Can you work these out from the model? Positions are in its coordinate system, mm. Face numbers are marked on the shaded views. A direction names the side the tool comes from. Give positions to 0.01 mm unless a question says otherwise; leave off trailing zeros. Loops run counter-clockwise (first coordinate to the right, second up) from the corner with the lowest first, then second, coordinate; pieces in that order, holes last. Notation, with made-up numbers: (69, 65) - (122, 65) arc R20 cw to (122, 90) - close; hole circle Ø5 at (51.5, 12.25). An arc over 180 degrees is marked (long way). Answer in a Markdown table with one row per item.
from build123d import *

# Parameters (mm, degrees)
SKETCH_1_R          = 14
EXTRUDE_1_DEPTH     = 22
SKETCH_2_R          = 2.95
CUT_EXTRUDE_1_DEPTH = 1.1
SKETCH_3_R          = 2.6
CUT_EXTRUDE_2_DEPTH = 9
SKETCH_5_R          = 6.1
CUT_EXTRUDE_3_DEPTH = 11.9
SKETCH_6_R          = 7.05
CUT_EXTRUDE_4_DEPTH = 7.9
SKETCH_7_R          = 7.6
CUT_EXTRUDE_5_DEPTH = 3.9
SKETCH_8_R          = 11.75
CUT_EXTRUDE_6_DEPTH = 1.9


with BuildPart() as part:
    # Эскиз1 → Бобышка-Вытянуть1 (new body)
    with BuildSketch(Plane.XY):
        Circle(SKETCH_1_R)
    extrude(amount=EXTRUDE_1_DEPTH)

    # Эскиз2 → Вырез-Вытянуть1 (cut)
    with BuildSketch(Plane(origin=(0, 0, 0), x_dir=(-1, 0, 0), z_dir=(0, 0, -1))):
        Circle(SKETCH_2_R)
    extrude(amount=-CUT_EXTRUDE_1_DEPTH, mode=Mode.SUBTRACT)

    # Эскиз3 → Вырез-Вытянуть2 (cut)
    with BuildSketch(Plane(origin=(0, 0, 1.1), x_dir=(-1, 0, 0), z_dir=(0, 0, -1))):
        Circle(SKETCH_3_R)
    extrude(amount=-CUT_EXTRUDE_2_DEPTH, mode=Mode.SUBTRACT)

    # Эскиз5 → Вырез-Вытянуть3 (cut)
    with BuildSketch(Plane.XY.offset(22)):
        Circle(SKETCH_5_R)
    extrude(amount=-CUT_EXTRUDE_3_DEPTH, mode=Mode.SUBTRACT)

    # Эскиз6 → Вырез-Вытянуть4 (cut)
    with BuildSketch(Plane.XY.offset(22)):
        Circle(SKETCH_6_R)
    extrude(amount=-CUT_EXTRUDE_4_DEPTH, mode=Mode.SUBTRACT)

    # Эскиз7 → Вырез-Вытянуть5 (cut)
    with BuildSketch(Plane.XY.offset(22)):
        Circle(SKETCH_7_R)
    extrude(amount=-CUT_EXTRUDE_5_DEPTH, mode=Mode.SUBTRACT)

    # Эскиз8 → Вырез-Вытянуть6 (cut)
    with BuildSketch(Plane.XY.offset(22)):
        Circle(SKETCH_8_R)
    extrude(amount=-CUT_EXTRUDE_6_DEPTH, mode=Mode.SUBTRACT)


solid = part.part
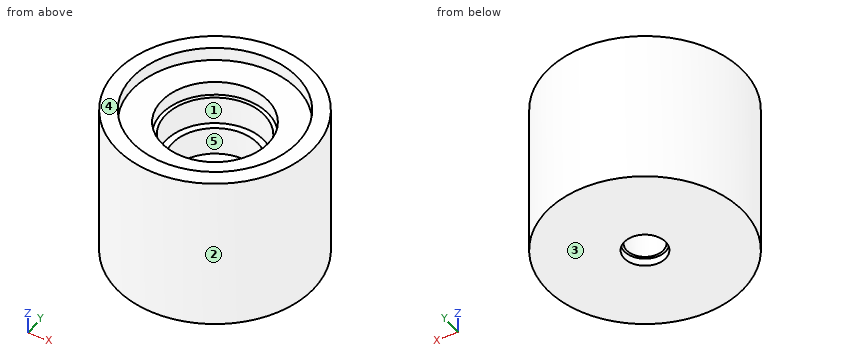
Q1. For pin 1 (7.5 mm diameter, centred on x = 1.5, y = -0.5, fed in from +Z); pin 2 (7 mm diameter, centred on x = -4.5, y = 3, fed in from +Z); pin 3 (6 mm diameter, centred on x = 11, z = 19, fed in from +Y), each with a flat end and sliding along its axis, tell me the tip position at first contact or that it passes through.
Checked values:
| item | result |
|---|---|
| pin 1 | stops at z = 10.1 |
| pin 2 | stops at z = 20.1 |
| pin 3 | stops at y = 11.49 |
Q2. If I drill on line 1 (Y direction, x = 0, z = 11.85); line 2 (Y direction, x = 0, z = 0.85); line 3 (Z direction, x = -4.25, y = -6.5), over which ranges is the centre line in solid material (lowest first)? Write a range as [from, to].
Checked values:
| item | result |
|---|---|
| line 1 | y = [-14, -6.1], [6.1, 14] |
| line 2 | y = [-14, -2.95], [2.95, 14] |
| line 3 | z = [0, 20.1] |
Q3. Imagine slicing it at C-C, the plane z = 20.5. Write out the boundary of the cut face in (x, y).
Checked values:
| item | result |
|---|---|
| outline | circle Ø28 at (0, 0); hole circle Ø23.5 at (0, 0) |
Q4. On a 3-axis mill with a long thin cutter (end or side, diameter ignored), from which of +Z, -Z, +X, -X, +Y, -Y can I reach the whole of each face in a straight line? I mean the marked faces 4 and 5. Say none if no direction works.
Checked values:
| item | result |
|---|---|
| face 4 | +Z, +X, -X, +Y, -Y |
| face 5 | +Z |
Q5. Imagine slicing it at D-D, the plane x = -11.25. Write out the boundary of the cut face in (y, z), and give its area (3 significant figures).
Checked values:
| item | result |
|---|---|
| outline | (-8.33, 0) - (8.33, 0) - (8.33, 22) - (3.39, 22) - (3.39, 20.1) - (-3.39, 20.1) - (-3.39, 22) - (-8.33, 22) - close |
| area | 354 mm² |
Q6. Imagine slicing it at A-A, the plane y = 0. Write out the boundary of the cut face in (x, z), and give its area (3 significant figures).
Checked values:
| item | result |
|---|---|
| outline | (-14, 0) - (-2.95, 0) - (-2.95, 1.1) - (-2.6, 1.1) - (-2.6, 10.1) - (-6.1, 10.1) - (-6.1, 14.1) - (-7.05, 14.1) - (-7.05, 18.1) - (-7.6, 18.1) - (-7.6, 20.1) - (-11.75, 20.1) - (-11.75, 22) - (-14, 22) - close; (2.6, 1.1) - (2.95, 1.1) - (2.95, 0) - (14, 0) - (14, 22) - (11.75, 22) - (11.75, 20.1) - (7.6, 20.1) - (7.6, 18.1) - (7.05, 18.1) - (7.05, 14.1) - (6.1, 14.1) - (6.1, 10.1) - (2.6, 10.1) - close |
| area | 382 mm² |
Q7. If we mould it in two halves opening along X, with no side actions, what happens to the marked faces 1, 2 and 3? For each: released by +X, released by -X, zero draft, split by the parting line, or undercut.
Checked values:
| item | result |
|---|---|
| face 1 | undercut |
| face 2 | split by the parting line |
| face 3 | zero draft |
